Check sheet for the modelled part. Datum: model origin and axes. Units: mm. Round coordinates to 2 decimals unless told otherwise and drop trailing zeros. Loops run counter-clockwise (first coordinate to the right, second up) from the corner with the lowest first, then second, coordinate; pieces in that order, holes last. Notation, with made-up numbers: (80.5, 63) -> (117.5, 63) arc R27 cw to (117.5, 96) -> close; hole circle Ø2 at (-33, 47.25). An arc over 180 degrees is marked (long way). One line per question, with ' | ' between items.
```python
from build123d import *

# Parameters (mm, degrees)
F0_W     = 834.740075
F0_H     = 50.8
F1_DEPTH = 3.048
F3_W     = 57.9247
F3_H     = 3.1496
F3_W_2   = 115.8494
F4_DEPTH = 3.048
F6_DEPTH = 3.048
F7_DEPTH = 3.049
F8_W     = 6.096
F8_H     = 6.096
F8_R     = 2.8702
F8_R_2   = 4.953
F8_R_3   = 7.9375
F9_DEPTH = 3.049


with BuildPart() as f1:
    # F0 (on Front) → F1 (new body)
    with BuildSketch(Plane.XZ):
        with Locations((417.370037, 25.4)):
            Rectangle(F0_W, F0_H)
    extrude(amount=F1_DEPTH)

    # F3 (on face) → F4 (join)
    with BuildSketch(Plane.XZ.offset(3.048)):
        with Locations((28.96235, 52.3748)):
            Rectangle(F3_W, F3_H)
        with Locations((139.123346, 52.3748)):
            Rectangle(F3_W_2, F3_H)
        with Locations((28.96235, -1.5748)):
            Rectangle(F3_W, F3_H)
        with Locations((139.123346, -1.5748)):
            Rectangle(F3_W_2, F3_H)
        with Locations((278.246692, 52.3748)):
            Rectangle(F3_W_2, F3_H)
        with Locations((278.246692, -1.5748)):
            Rectangle(F3_W_2, F3_H)
        with Locations((417.370038, 52.3748)):
            Rectangle(F3_W_2, F3_H)
        with Locations((417.370038, -1.5748)):
            Rectangle(F3_W_2, F3_H)
        with Locations((556.493384, 52.3748)):
            Rectangle(F3_W_2, F3_H)
        with Locations((556.493384, -1.5748)):
            Rectangle(F3_W_2, F3_H)
        with Locations((695.61673, 52.3748)):
            Rectangle(F3_W_2, F3_H)
        with Locations((695.61673, -1.5748)):
            Rectangle(F3_W_2, F3_H)
        with Locations((805.777725, 52.3748)):
            Rectangle(F3_W, F3_H)
        with Locations((805.777725, -1.5748)):
            Rectangle(F3_W, F3_H)
    extrude(amount=-F4_DEPTH)

    # F5 (on face) → F6 (join)
    with BuildSketch(Plane.XZ.offset(3.048)):
        Polygon((-6.35, 6.35), (0, 6.35), (0, 44.45), (-6.35, 44.45), (-9.525, 47.625), (-9.525, 3.175), align=None)
    extrude(amount=-F6_DEPTH)

    # F5 (on face) → F7 (cut, through all)
    with BuildSketch(Plane.XZ.offset(3.048)):
        Polygon((828.390075, 6.35), (834.740075, 6.35), (834.740075, 44.45), (828.390075, 44.45), (825.215075, 47.625), (825.215075, 3.175), align=None)
    extrude(amount=-F7_DEPTH, mode=Mode.SUBTRACT)

    # F8 (on face) → F9 (cut, through all)
    with BuildSketch(Plane.XZ.offset(3.048)):
        with Locations((256.326492, 15.5194)):
            Rectangle(F8_W, F8_H)
        with Locations((278.246692, 15.5194)):
            Rectangle(F8_W, F8_H)
        with Locations((300.166892, 15.5194)):
            Rectangle(F8_W, F8_H)
        with Locations((235.701692, 15.5194)):
            Circle(F8_R)
        with Locations((323.966692, 15.5194)):
            Circle(F8_R_2)
        with Locations((278.246692, 34.5694)):
            Circle(F8_R_3)
    extrude(amount=-F9_DEPTH, mode=Mode.SUBTRACT)


solid = f1.part
```
(1) Sectioned sample at B-B, the plane y = -0.6. Count the separate pieces of the cut face and the enclosed holes in it, and give its area (3 significant figures).
Answer:
separate pieces: 1 | enclosed holes: 6 | area: 46,400 mm2
(2) Scan lines: probe 1 along X at (y, z) = (-1.55, 16.5) (1 decimal); probe 2 along X at (y, z) = (-0.4, 3.5) (3 decimals); probe 3 along X at (y, z) = (-1.65, 48.5). Record each from-to range of solid material in increasing order.
Answer:
probe 1: x = -9.5 to 233, 238.4 to 253.3, 259.4 to 275.2, 281.3 to 297.1, 303.2 to 319.1, 328.8 to 825.2 | probe 2: x = -9.525 to -9.2, 0 to 825.215, 825.54 to 834.74 | probe 3: x = 0 to 834.74
(3) Sectioned sample at A-A, the plane x = 205.5. Record the cut outline in (y, z).
Answer:
outline: (-3.05, 0) -> (0, 0) -> (0, 50.8) -> (-3.05, 50.8) -> close
(4) Go/stop test with flat-tipped pins: pin 1 (0.9 mm diameter, centred on y = -1, z = -2.5, fed in from -X); pin 2 (0.9 mm diameter, centred on x = 348, y = -2, fed in from -Z). Record where each tip stops, or that it passes through.
Answer:
pin 1: stops at x = 0 | pin 2: stops at z = 0
